Input: part model. Units: mm. Frame: model coordinates. A direction names the side the tool comes from. Coordinates: 2 decimals unless noted, no trailing zeros. Write each loop counter-clockwise with the first axis right and the second up, starting at its lowest first coordinate (ties: lowest second). Pieces come first, ordered by that corner, then holes. Notation, with made-up numbers: (-33, -34) - (13, -34) arc R23 ccw to (13, -11) - close; hole circle Ø2 at (26.25, -22.5). An arc over 180 degrees is marked (long way). Use CSV: the item, a comma, the result in double quotes.
```python
from build123d import *

# Parameters (mm, degrees)
SKETCH1_W          = 10
SKETCH1_H          = 1.5
CHAMFER1_SIZE      = 0.375
CUT_EXTRUDE2_DEPTH = 1.155


with BuildPart() as part:
    # Sketch1 → Revolve1 (revolve)
    with BuildSketch(Plane(origin=(0, 0, 0), x_dir=(0, 0, -1), z_dir=(1, 0, 0))):
        with Locations((6.65, 0.75)):
            Rectangle(SKETCH1_W, SKETCH1_H)
    revolve(axis=Axis((0, 0, -11.65), (0, 0, 1)))

    # Chamfer1
    chamfer1_edges = [part.edges().sort_by_distance(p)[0] for p in [
        (0, -1.5, -11.65),
    ]]
    chamfer(chamfer1_edges, length=CHAMFER1_SIZE)

    # Sketch7 → Revolve2 (revolve)
    with BuildSketch(Plane(origin=(0, 0, 0), x_dir=(0, 0, -1), z_dir=(1, 0, 0)), mode=Mode.PRIVATE) as revolve2_sk:
        with BuildLine():
            Line((1.4025, 2.85), (1.65, 2.85))
            Line((1.65, 2.85), (1.65, 0))
            Line((1.65, 0), (0, 0))
            Line((0, 0), (0, 1.5))
            ThreePointArc((0, 1.5), (0.59512511, 2.285251969), (1.4025, 2.85))
        make_face()
    revolve(revolve2_sk.sketch.rotate(Axis((0, 0, 0), (0, 0, -1)), 180), axis=Axis((0, 0, 0), (0, 0, -1)))

    # Sketch5 → Cut-Extrude2 (cut)
    with BuildSketch(Plane.XY):
        Polygon((1, -0.577350269), (1, 0.577350269), (0, 1.154700538), (-1, 0.577350269), (-1, -0.577350269), (0, -1.154700538), align=None)
    extrude(amount=-CUT_EXTRUDE2_DEPTH, mode=Mode.SUBTRACT)


solid = part.part
```
(1) Cut plane C-C on y = 2.2. Return loops of the section in (x, z).
Check values:
outline,"(-1.81, -1.65) - (1.81, -1.65) - (1.81, -1.4) arc R2.28 ccw to (-1.81, -1.4) - close"
(2) Ray query, probe 1 along Z at (x, y) = (0.6, 0.75) (3 decimals); probe 2 along Y at (x, z) = (0.05, -4.75). Return the intervals inside material, ascending. Write a range as from..to.
Check values:
probe 1,"-11.65..-1.155"
probe 2,"-1.5..1.5"
(3) Cut plane B-B on z = -7.25. Return loops of the section in (x, y).
Check values:
outline,"circle Ø3 at (0, 0)"
(4) Draft query along Y for faces 3 (the flat face through (0.51, 0.86, -0.57)), 4 (the cylindrical face through (-0.07, -1.5, -6.53)), 5 (the flat face through (0, 0, -11.65)), 6 (the flat face through (-0.49, 0.87, -0.57)). Return one class per face: pulls with the +Y half, pulls with the -Y half, needs draft (parallel to the pull), parting line crosses it, or undercut.
Check values:
face 3,"undercut"
face 4,"parting line crosses it"
face 5,"needs draft"
face 6,"undercut"
(5) Reachability of faces 1 (the flat face through (1.2, -1.2, -1.65)), 2 (the flat face through (-1, 0, -1)) from +Z, -Z, +X, -X, +Y, -Y: full face, straight path, thin tool, end or side. Return the list, or none.
Check values:
face 1,"-Z"
face 2,"+Z"
(6) Pin query (flat end, axial travel): pin 1 Ø2 at (x, z) = (-1.5, -6) entering from -Y; pin 2 Ø1.3 at (y, z) = (0, -0.5) entering from -X. Return the tip coordinate at first contact, or that it passes through.
Check values:
pin 1,"y = -1.41"
pin 2,"x = -2.71"
